Could you check a few things on this model? Use its own coordinates, in mm. A direction names the side the tool comes from. Give positions to 0.01 mm unless a question says otherwise; leave off trailing zeros. Loops run counter-clockwise (first coordinate to the right, second up) from the corner with the lowest first, then second, coordinate; pieces in that order, holes last.
1. Imagine slicing it at A-A (z = 0). List the corners of the cut face in (x, y) for me, plus the area to 3 significant figures.
2. For faces 1 (the cylindrical face through (-10.352, 0.33, -7.493)), 2 (the flat face through (-0.5, -0.2, -0.5)), 3 (the flat face through (0, 0, 6)), which set-ups out of +Z, -Z, +X, -X, +Y, -Y let a thin tool reach every point of the face, with its end or its side?
3. For P1, Ø1.5, axis at x = -8, y = 1, coming from the +Z side; P2, Ø10, axis at y = -4.5, z = -10.5, coming from the -X side; P3, Ø10, axis at x = -9.5, z = -7, coming from the +Y side; P4, Ø10, axis at x = -7.5, z = 7.5, coming from the +Y side, each with a flat end and sliding along its axis, tell me the tip position at first contact or that it passes through.
4. Imagine slicing it at D-D (y = -8.5). List the corners of the cut face in (x, z) for me.
5. Imagine slicing it at C-C (x = -4.75). List the corners of the cut face in (y, z) for me.
6. Imagine slicing it at B-B (y = 0). List the corners of the cut face in (x, z) for me, plus the area to 3 significant figures.
7. I need wall thicknesses on line 1 along X through (y, z) = (9, 3.25); line 2 along Z through (x, y) = (-5.5, -1.25); line 3 along Y through (x, z) = (-16.75, -5). Which ranges of each line are inside material? Lowest first, please.
8. Thinking about a two-plate mould opening in Z: for faces 4 (the flat face through (-1, 0, 0)), 5 (the flat face through (-0.5, 0.2, 0.5)), 6 (the flat face through (-18, 0, 0)), 7 (the cylindrical face through (-1.521, 0.66, -14.985)), which applies, +Z half, -Z half, draft (parallel to the pull), parting line (faces both ways), or undercut?
Autodesk Inventor part; units mm, degrees
ref_plane "YZ Plane" through (0, 0, 0) normal (1, 0, 0) x (0, 1, 0)
ref_plane "XZ Plane" through (0, 0, 0) normal (0, 1, 0) x (-1, 0, 0)
ref_plane "XY Plane" through (0, 0, 0) normal (0, 0, 1) x (1, 0, 0)
sketch "Эскиз1" plane through (0, 0, 0) normal (0, 1, 0) x (-1, 0, 0)
  line L0 (0, 0) -> (0, 15)
  line L1 (0, 15) -> (3, 15)
  line L2 (0, 0) -> (3, 0)
  line L3 (3, 0) -> (18, 0)
  line L4 (18, 0) -> (18, 7.5)
  line L5 (18, 7.5) -> (6, 7.5)
  line L6 (3, 7.5) -> (3, 15)
  line L7 (3, 15) -> (3, 7.5)
  line L8 (3, 7.5) -> (6, 7.5)
  line L9 (6, 7.5) -> (6, 7.5)
  dimension "d0" = 15
  dimension "d1" = 3
  dimension "d2" = 15
  dimension "d3" = 7.5
  dimension "d4" = 7.5
  dimension "d5" = 3
revolve "Вращение1" add sketch "Эскиз1" angle 360 about axis through (-3, 0, 0) along (-1, 0, 0)
thread "Резьба1"
chamfer "Фаска1" distance 0.5 angle 45 1 edges at (-18, 0, -7.5)
sketch "Эскиз2" plane through (0, 0, 0) normal (1, 0, 0) x (0, 0, -1)
  line L0 (0, 0) -> (-0.5, 0)
  line L1 (-0.5, 0) -> (-0.5, -15.5387)
  line L2 (-0.5, -15.5387) -> (0.5, -15.5387)
  line L3 (0.5, -15.5387) -> (0.5, 16.3638)
  line L4 (0.5, 16.3638) -> (-0.5, 16.3638)
  line L5 (-0.5, 16.3638) -> (-0.5, -15.5387)
  dimension "d12" = 0.5
  dimension "d13" = 1
extrude "Выдавливание1" cut sketch "Эскиз2" against normal blind 1
properties part number "Болт М15х1,5"
Derived:
1. outline: (-18, -7) - (-17.5, -7.5) - (-3, -7.5) - (-3, -15) - (-1, -15) - (-1, 15) - (-3, 15) - (-3, 7.5) - (-17.5, 7.5) - (-18, 7) - close
1. area: 285 mm2
2. face 1: -X
2. face 2: +X, +Y, -Y
2. face 3: +Z, -Z, +X, +Y, -Y
3. P1: stops at z = 7.5
3. P2: stops at x = -18
3. P3: stops at y = 7.23
3. P4: stops at y = 14.02
4. outline: (-3, -12.36) - (0, -12.36) - (0, -0.5) - (-1, -0.5) - (-1, 0.5) - (0, 0.5) - (0, 12.36) - (-3, 12.36) - close
5. outline: circle Ø15 at (0, 0)
6. outline: (-18, -7) - (-17.5, -7.5) - (-3, -7.5) - (-3, -15) - (0, -15) - (0, -0.5) - (-1, -0.5) - (-1, 0.5) - (0, 0.5) - (0, 15) - (-3, 15) - (-3, 7.5) - (-17.5, 7.5) - (-18, 7) - close
6. area: 314 mm2
7. line 1: x = -3 to 0
7. line 2: z = -7.4 to 7.4
7. line 3: y = -5.59 to 5.59
8. face 4: undercut
8. face 5: undercut
8. face 6: draft
8. face 7: parting line
